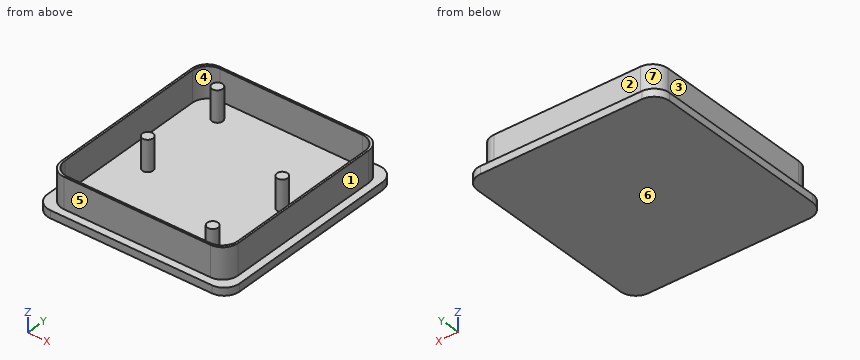
from build123d import *

# Parameters (mm, degrees)
BOSS_EXTRUDE1_DEPTH = 10
SKETCH3_R           = 1.4
CUT_EXTRUDE2_DEPTH  = 8


with BuildPart() as part:
    # Sketch1 → Boss-Extrude1 (new body)
    with BuildSketch(Plane.XY):
        with BuildLine():
            Line((-21, -27), (21, -27))
            ThreePointArc((21, -27), (23.828427125, -25.828427125), (25, -23))
            Line((25, -23), (25, 23))
            ThreePointArc((25, 23), (23.828427125, 25.828427125), (21, 27))
            Line((21, 27), (-21, 27))
            ThreePointArc((-21, 27), (-23.828427125, 25.828427125), (-25, 23))
            Line((-25, 23), (-25, -23))
            ThreePointArc((-25, -23), (-23.828427125, -25.828427125), (-21, -27))
        make_face()
    extrude(amount=BOSS_EXTRUDE1_DEPTH)

    # Sketch3 → Cut-Extrude2 (cut)
    with BuildSketch(Plane.XY.offset(10)):
        with BuildLine():
            Line((21, 27), (-21, 27))
            ThreePointArc((-21, 27), (-23.828427125, 25.828427125), (-25, 23))
            Line((-25, 23), (-25, -23))
            ThreePointArc((-25, -23), (-23.828427125, -25.828427125), (-21, -27))
            Line((-21, -27), (21, -27))
            ThreePointArc((21, -27), (23.828427125, -25.828427125), (25, -23))
            Line((25, -23), (25, 23))
            ThreePointArc((25, 23), (23.828427125, 25.828427125), (21, 27))
        make_face()
        with BuildLine():
            Line((-19, -25), (19, -25))
            ThreePointArc((19, -25), (21.828427125, -23.828427125), (23, -21))
            Line((23, -21), (23, 21))
            ThreePointArc((23, 21), (21.828427125, 23.828427125), (19, 25))
            Line((19, 25), (-19, 25))
            ThreePointArc((-19, 25), (-21.828427125, 23.828427125), (-23, 21))
            Line((-23, 21), (-23, -21))
            ThreePointArc((-23, -21), (-21.828427125, -23.828427125), (-19, -25))
        make_face(mode=Mode.SUBTRACT)
        with BuildLine():
            Line((-18.5, -24.5), (18.5, -24.5))
            ThreePointArc((18.5, -24.5), (21.328427125, -23.328427125), (22.5, -20.5))
            Line((22.5, -20.5), (22.5, 20.5))
            ThreePointArc((22.5, 20.5), (21.328427125, 23.328427125), (18.5, 24.5))
            Line((18.5, 24.5), (-18.5, 24.5))
            ThreePointArc((-18.5, 24.5), (-21.328427125, 23.328427125), (-22.5, 20.5))
            Line((-22.5, 20.5), (-22.5, -20.5))
            ThreePointArc((-22.5, -20.5), (-21.328427125, -23.328427125), (-18.5, -24.5))
        make_face()
        with Locations((-15, -3.1)):
            Circle(SKETCH3_R, mode=Mode.SUBTRACT)
        with Locations((15, 3.1)):
            Circle(SKETCH3_R, mode=Mode.SUBTRACT)
        with Locations((-15, 19.3)):
            Circle(SKETCH3_R, mode=Mode.SUBTRACT)
        with Locations((15, -19.3)):
            Circle(SKETCH3_R, mode=Mode.SUBTRACT)
    extrude(amount=-CUT_EXTRUDE2_DEPTH, mode=Mode.SUBTRACT)


solid = part.part
Source: CAD feature listing. Evaluate the final solid. Frame: model axes, mm. Face numbers are marked on the shaded views. A direction names the side the tool comes from. Coordinates: 2 decimals unless noted, no trailing zeros. Loops run counter-clockwise (first coordinate to the right, second up) from the corner with the lowest first, then second, coordinate; pieces in that order, holes last. Notation, with made-up numbers: (-12, 13) -> (38, 13) arc R24 ccw to (38, 27) -> close; hole circle Ø5 at (-18, 16). An arc over 180 degrees is marked (long way). Answer in a Markdown table with one row per item. Add a question column.
Q1. Pull-direction query (Y, two-part tool) for the marked faces 4, 5, 6 and 7; classes: pulls with the +Y half, pulls with the -Y half, needs draft (parallel to the pull), parting line crosses it, or undercut.
Q2. Section C-C on x = -4.5. Return the cut outline in (y, z).
Q3. Contact query for flat-ended pins moving along their axis: pin 1 Ø6 at (y, z) = (12, 9) entering from -X; pin 2 Ø2.5 at (y, z) = (9, 6) entering from +X; pin 3 Ø1.5 at (x, z) = (-9, 3) entering from -Y. Output: stop coordinate, or through.
Q4. Section D-D on y = -11. Return the cut outline in (x, z).
Q5. Section B-B on y = -19.3. Return the cut outline in (x, z), and give its area (3 significant figures).
Q6. Reachability of the marked faces 1, 2 and 3 from +Z, -Z, +X, -X, +Y, -Y: full face, straight path, thin tool, end or side. Return the list, or none.
Q7. Ray query, line 1 along Y through (x, z) = (18.5, 2.75); line 2 along X through (y, z) = (-15, 6.25); line 3 along Y through (x, z) = (-14, 8). Return the intervals inside material, ascending.
Q8. Section A-A on z = 7.5. Return the cut outline in (x, y).
Computed values:
| question | item | result |
|---|---|---|
| 1 | face 4 | undercut |
| 1 | face 5 | pulls with the -Y half |
| 1 | face 6 | needs draft |
| 1 | face 7 | pulls with the +Y half |
| 2 | outline | (-27, 0) -> (27, 0) -> (27, 2) -> (25, 2) -> (25, 10) -> (24.5, 10) -> (24.5, 2) -> (-24.5, 2) -> (-24.5, 10) -> (-25, 10) -> (-25, 2) -> (-27, 2) -> close |
| 3 | pin 1 | stops at x = -23 |
| 3 | pin 2 | stops at x = 23 |
| 3 | pin 3 | stops at y = -25 |
| 4 | outline | (-25, 0) -> (25, 0) -> (25, 2) -> (23, 2) -> (23, 10) -> (22.5, 10) -> (22.5, 2) -> (-22.5, 2) -> (-22.5, 10) -> (-23, 10) -> (-23, 2) -> (-25, 2) -> close |
| 5 | outline | (-25, 0) -> (25, 0) -> (25, 2) -> (23, 2) -> (23, 10) -> (22.5, 10) -> (22.5, 2) -> (16.4, 2) -> (16.4, 10) -> (13.6, 10) -> (13.6, 2) -> (-22.5, 2) -> (-22.5, 10) -> (-23, 10) -> (-23, 2) -> (-25, 2) -> close |
| 5 | area | 130 mm^2 |
| 6 | face 1 | +Z, +X, +Y, -Y |
| 6 | face 2 | +Z, +X, -X, +Y |
| 6 | face 3 | +Z, -X, +Y, -Y |
| 7 | line 1 | y = -25 to -24.5, 24.5 to 25 |
| 7 | line 2 | x = -23 to -22.5, 22.5 to 23 |
| 7 | line 3 | y = -25 to -24.5, -4.08 to -2.12, 18.32 to 20.28, 24.5 to 25 |
| 8 | outline | (-23, -21) arc R4 ccw to (-19, -25) -> (19, -25) arc R4 ccw to (23, -21) -> (23, 21) arc R4 ccw to (19, 25) -> (-19, 25) arc R4 ccw to (-23, 21) -> close; circle Ø2.8 at (-15, -3.1); circle Ø2.8 at (-15, 19.3); circle Ø2.8 at (15, -19.3); circle Ø2.8 at (15, 3.1); hole (-22.5, -20.5) arc R4 ccw to (-18.5, -24.5) -> (18.5, -24.5) arc R4 ccw to (22.5, -20.5) -> (22.5, 20.5) arc R4 ccw to (18.5, 24.5) -> (-18.5, 24.5) arc R4 ccw to (-22.5, 20.5) -> close |
